Autodesk Inventor part; units mm, degrees
ref_plane "YZ Plane" through (0, 0, 0) normal (1, 0, 0) x (0, 1, 0)
ref_plane "XZ Plane" through (0, 0, 0) normal (0, 1, 0) x (-1, 0, 0)
ref_plane "XY Plane" through (0, 0, 0) normal (0, 0, 1) x (1, 0, 0)
sketch "Sketch1" plane through (0, 0, 0) normal (0, 0, 1) x (1, 0, 0)
  line L0 (0, 0) -> (0, 25.4)
  arc A0 (0, 25.4) -> (-25.4, 50.8) centre (-25.4, 25.4) ccw
  line L1 (-25.4, 50.8) -> (-50.8, 50.8)
  arc A1 (-50.8, 50.8) -> (-76.2, 25.4) centre (-50.8, 25.4) ccw
  line L2 (-76.2, 25.4) -> (-76.2, 0)
  line L3 (-76.2, 0) -> (0, 0)
  point P0 (-38.1, 12.7)
extrude "Extrusion1" add sketch "Sketch1" along normal blind 25.4
hole "Hole1" at (-38.1, 12.7, 0) direction (0, 0, 1) diameter 3.9624 depth 12.7 tip angle 118
properties part number "arc_test"
Input: part model. Units: mm. Frame: model coordinates. Coordinates: 2 decimals unless noted, no trailing zeros. Write each loop counter-clockwise with the first axis right and the second up, starting at its lowest first coordinate (ties: lowest second). Pieces come first, ordered by that corner, then holes. Notation, with made-up numbers: (42.25, 39.25) -> (95.25, 39.25) arc R18 ccw to (95.25, 73.25) -> close; hole circle Ø4 at (-38.75, 88). An arc over 180 degrees is marked (long way). Write each question's results on one line, items separated by ' | '.
Item 1: Section query A-A on z = 4.5. Return loops of the section in (x, y), plus the area to 3 significant figures.
Conclusion:
outline: (-76.2, 0) -> (0, 0) -> (0, 25.4) arc R25.4 ccw to (-25.4, 50.8) -> (-50.8, 50.8) arc R25.4 ccw to (-76.2, 25.4) -> close; hole circle Ø3.96 at (-38.1, 12.7) | area: 3,580 mm^2
Item 2: Section query D-D on x = -59. Return loops of the section in (y, z).
Conclusion:
outline: (0, 0) -> (49.44, 0) -> (49.44, 25.4) -> (0, 25.4) -> close
Item 3: Material intervals for probe 1 along X at (y, z) = (12.7, 6.25); probe 2 along Y at (x, z) = (-38.1, 7); probe 3 along X at (y, z) = (29, 9), sorted ascending.
Conclusion:
probe 1: x = -76.2 to -40.08, -36.12 to 0 | probe 2: y = 0 to 10.72, 14.68 to 50.8 | probe 3: x = -75.94 to -0.26
Item 4: Mould query, pull axis X, two halves, no side actions, for faces 1 (the flat face through (-76.2, 13, 13)), 2 (the cylindrical face through (-39.771, 13.765, 6.439)), 3 (the flat face through (-39, 0, 13)), 4 (the flat face through (0, 13, 13)). Classes: +X half, -X half, draft (parallel to the pull), parting line (faces both ways), or undercut.
Conclusion:
face 1: -X half | face 2: undercut | face 3: draft | face 4: +X half
Item 5: Section query C-C on x = -14. Return loops of the section in (y, z), plus the area to 3 significant figures.
Conclusion:
outline: (0, 0) -> (48.1, 0) -> (48.1, 25.4) -> (0, 25.4) -> close | area: 1,220 mm^2
Item 6: Section query B-B on z = 21.5. Return loops of the section in (x, y).
Conclusion:
outline: (-76.2, 0) -> (0, 0) -> (0, 25.4) arc R25.4 ccw to (-25.4, 50.8) -> (-50.8, 50.8) arc R25.4 ccw to (-76.2, 25.4) -> close
